Read the model definition and answer for the solid it produces. Units are mm, in the model's axes. A direction names the side the tool comes from. Give positions to 0.01 mm unless a question says otherwise; leave off trailing zeros. Loops run counter-clockwise (first coordinate to the right, second up) from the corner with the lowest first, then second, coordinate; pieces in that order, holes last. Notation, with made-up numbers: (68, -8) -> (81, -8) arc R25 ccw to (81, 23) -> close; hole circle Ø3 at (9.5, 50.5). An arc over 180 degrees is marked (long way). Write each question's results on one line, items separated by ' | '. Start each with the question number.
Item 1: Which of the six approach directions +Z, -Z, +X, -X, +Y, -Y give full straight-line access (tool end or side, diameter ignored) to faces 1 (the flat face through (69, -35, 1)), 2 (the flat face through (73, -4, 14)), 3 (the flat face through (69, 35, 1)), 4 (the flat face through (67, -4, 19))?
Item 2: Section C-C on z = 13.5 is taken. Write down the section's boundary in (x, y), and give its area (3 significant figures).
Item 3: Section B-B on y = -7 is taken. State how many separate pieces and enclosed holes the cut face has, and give its area (3 significant figures).
Item 4: Find the intervals of material crossed by line 1 (Y direction, x = 0, z = -0.05); line 2 (Z direction, x = 70, y = -7); line 3 (Z direction, x = 50.5, y = -52), in increasing order.
Item 5: Section A-A on z = 30 is taken. Write down the section's boundary in (x, y), and give its area (3 significant figures).
Item 6: Each of these flat-tipped pins is pushed along its axis until it touches: P1, Ø2.5, axis at x = 70.5, z = 1, coming from the -Y side; P2, Ø8, axis at y = 2.5, z = 16.5, coming from the -X side; P3, Ø1.5, axis at x = 68, z = 1.5, coming from the +Y side. Where does it stop, or does it pass through?
Item 7: Determine the mould class of faces 5 (the cylindrical face through (69.293, 60.091, -0.158)), 6 (the flat face through (70, -7, 44)), 7 (the cylindrical face through (70.042, -9.428, 19.066)) for opening direction Y: +Y half, -Y half, draft (parallel to the pull), parting line (faces both ways), or undercut.
```python
from build123d import *

# Parameters (mm, degrees)
SKETCH001_R     = 45
PAD_DEPTH       = 1.12
SKETCH_W        = 8
SKETCH_H        = 70
PAD003_DEPTH    = 3
SKETCH008_W     = 6
SKETCH008_H     = 30
PAD004_DEPTH    = 41
SKETCH009_R     = 11.2
POCKET003_DEPTH = 137.0009178097
POCKET004_DEPTH = 137.0009178097
FILLET_R        = 0.8


with BuildPart() as part:
    # Sketch001 → Pad (new body)
    with BuildSketch(Plane.XY):
        with BuildLine():
            Line((60, 64), (0, 64))
            ThreePointArc((0, 63.9999999999), (-63.9999178097, 0), (0, -63.9999999999))
            Line((60, -63.9999999999), (0, -63.9999999999))
            ThreePointArc((60, -64), (69.1923881554, -60.1923881554), (73, -51))
            Line((73, 51), (73, -51))
            ThreePointArc((73, 51), (69.1923881554, 60.1923881554), (60, 64))
        make_face()
        Circle(SKETCH001_R, mode=Mode.SUBTRACT)
    extrude(amount=-PAD_DEPTH)

    # Sketch → Pad003 (new body)
    with BuildSketch(Plane.XY):
        with Locations((69, 0)):
            Rectangle(SKETCH_W, SKETCH_H)
    extrude(amount=PAD003_DEPTH)

    # Sketch008 → Pad004 (new body)
    with BuildSketch(Plane.XY.offset(3)):
        with Locations((70, -7)):
            Rectangle(SKETCH008_W, SKETCH008_H)
    extrude(amount=PAD004_DEPTH)

    # Sketch009 → Pocket003 (cut, through all)
    with BuildSketch(Plane.YZ.offset(73)):
        with Locations((-7, 30)):
            Circle(SKETCH009_R)
    extrude(amount=-POCKET003_DEPTH, mode=Mode.SUBTRACT)

    # Sketch010 → Pocket004 (cut, through all)
    with BuildSketch(Plane.YZ.offset(73)):
        Polygon((-7, 48), (15, 36), (15, 54.3744), (-29, 54.3744), (-29, 36), align=None)
    extrude(amount=-POCKET004_DEPTH, mode=Mode.SUBTRACT)

    # Fillet
    fillet_edges = [part.edges().sort_by_distance(p)[0] for p in [
        (69.192388, 60.192388, -1.12),
        (30, 64, -1.12),
        (-63.999918, 0, -1.12),
        (30, -64, -1.12),
        (69.192388, -60.192388, -1.12),
        (73, 0, -1.12),
        (-45, 0, -1.12),
    ]]
    fillet(fillet_edges, radius=FILLET_R)


solid = part.part
```
Findings:
1) face 1: +Z, +X, -X, -Y | face 2: +Z, -Z, +X, +Y, -Y | face 3: +Z, +X, -X, +Y | face 4: +Z, -X, +Y, -Y
2) outline: (67, -22) -> (73, -22) -> (73, 8) -> (67, 8) -> close | area: 180 mm2
3) separate pieces: 3 | enclosed holes: 0 | area: 188 mm2
4) line 1: -64 to -45, 45 to 64 | line 2: -1.12 to 18.8, 41.2 to 44 | line 3: -1.12 to 0
5) outline: (67, -22) -> (73, -22) -> (73, -18.2) -> (67, -18.2) -> close; (67, 4.2) -> (73, 4.2) -> (73, 8) -> (67, 8) -> close | area: 45.6 mm2
6) P1: y = -59.6 | P2: x = 67 | P3: y = 35
7) face 5: +Y half | face 6: draft | face 7: undercut
